Design review of the part built by this model. Coordinates are the model's own, in mm. A direction names the side the tool comes from. Round coordinates to 2 decimals unless told otherwise and drop trailing zeros. Loops run counter-clockwise (first coordinate to the right, second up) from the corner with the lowest first, then second, coordinate; pieces in that order, holes last. Notation, with made-up numbers: (18, -34.5) - (43, -34.5) arc R37 cw to (43, 3.5) - close; hole circle Ø4 at (-25, 10). An arc over 180 degrees is marked (long way). Return JSON: item names as keys, results as strings. Group by question number.
from build123d import *

# Parameters (mm, degrees)
F1_DEPTH = 82.296
F3_DEPTH = 17.018
F4_DEPTH = 13.462


with BuildPart() as f1:
    # F0 (on Front) → F1 (new body)
    with BuildSketch(Plane.XZ):
        Polygon((-19.499537, 41.320443), (-54.165378, 41.320443), (-53.855862, 34.201566), (-20.428086, 34.201566), (-20.428086, 18.106712), (-20.428086, -2.63089), (34.975354, -2.63089), (34.975354, 9.749768), (-6.190328, 9.749768), (-6.190328, 41.320443), align=None)
    extrude(amount=F1_DEPTH)

    # F2 (on Front) → F3 (join)
    with BuildSketch(Plane.XZ):
        Polygon((13.618723, 41.320443), (-6.499845, 41.320443), (-5.880812, 10.678317), (13.618723, 10.678317), align=None)
    extrude(amount=F3_DEPTH)

    # F3_face (on face) → F4 (join)
    with BuildSketch(Plane(origin=(3.752634, -17.018, 26.039435), x_dir=(1, 0, 0), z_dir=(0, -1, 0))):
        Polygon((-9.942962, -0.040067), (-9.633446, -15.361118), (9.866089, -15.361118), (9.866089, 15.281008), (-9.942962, 15.281008), align=None)
    extrude(amount=F4_DEPTH)


solid = f1.part
Q1. Add section C-C, the plane y = -20.5. State the section outline as (x, z) points, plus the area to 3 significant figures.
Q2. Draft analysis for pull direction Z (two halves, no side actions). For faces 4 (the flat face through (-10, 0, 20)), 5 (the flat face through (-27, -41, 41.32)), 6 (the flat face through (15, -41, 9.75)), state which applies: pulls with the +Z half, pulls with the -Z half, needs draft (parallel to the pull), parting line crosses it, or undercut.
Q3. For line 1 (Z direction, x = -2, y = -6.5); line 2 (X direction, y = -33.5, z = 15); line 3 (Z direction, x = -49, y = -29), list the stretches that pass through material, from the lowest coordinate up.
Q4. Add section A-A, the plane x = 5. State the section outline as (y, z) points, plus the area to 3 significant figures.
Q5. Add section D-D, the plane z = 28.5. State the section outline as (x, y) points.
Q6. Tool access review of faces 1 (the flat face through (4, -15, 10.678)), 2 (the flat face through (-37, -41, 34.202)), 3 (the flat face through (4, -30.48, 26)): name each direction out of +Z, -Z, +X, -X, +Y, -Y from which nothing blocks a thin tool from reaching the whole face with its end or side.
Q7. Insertion check: pin 1 Ø8 at (y, z) = (-21.5, 9.5) entering from -X; pin 2 Ø6 at (y, z) = (-18.5, 32.5) entering from -X; pin 3 Ø10 at (x, y) = (-33, -57) entering from -Z. Each pin has a flat end and moves straight along its axis. Give the tip position at first contact, or say it passes through.
Q8. Add section B-B, the plane z = 19. State the section outline as (x, y) points.
Evaluation:
{
 "1": {"outline": "(-54.17, 41.32) - (-53.86, 34.2) - (-20.43, 34.2) - (-20.43, -2.63) - (34.98, -2.63) - (34.98, 9.75) - (-6.19, 9.75) - (-6.19, 26) - (-5.88, 10.68) - (13.62, 10.68) - (13.62, 41.32) - close", "area": "1,980 mm²"},
 "2": {"face 4": "needs draft", "face 5": "pulls with the +Z half", "face 6": "undercut"},
 "3": {"line 1": "-2.63 to 9.75, 10.68 to 41.32", "line 2": "-20.43 to -6.19", "line 3": "34.2 to 41.32"},
 "4": {"outline": "(-82.3, -2.63) - (0, -2.63) - (0, 9.75) - (-82.3, 9.75) - close; (-30.48, 10.68) - (0, 10.68) - (0, 41.32) - (-30.48, 41.32) - close", "area": "1,950 mm²"},
 "5": {"outline": "(-20.43, -82.3) - (-6.19, -82.3) - (-6.19, -30.48) - (13.62, -30.48) - (13.62, 0) - (-20.43, 0) - close"},
 "6": {"face 1": "+X, +Y, -Y", "face 2": "-Z, -X, +Y, -Y", "face 3": "+Z, +X, -Y"},
 "7": {"pin 1": "x = -20.43", "pin 2": "x = -53.91", "pin 3": "z = 34.2"},
 "8": {"outline": "(-20.43, -82.3) - (-6.19, -82.3) - (-6.19, 0) - (-20.43, 0) - close; (-6.05, -30.48) - (13.62, -30.48) - (13.62, 0) - (-6.05, 0) - close"}
}
